Job drawing, mm, ordinate dimensions from the low corner. One solid piece. A direction names the side the tool comes from. Give positions to 0.01 mm unless a question says otherwise; leave off trailing zeros. Order: outer loops, then holes, each group sorted by start corner. A loop starts at its lowest first (then second) coordinate and runs counter-clockwise, first axis right, second up. Notation, with made-up numbers: (-31.5, 31) -> (-0.5, 31) arc R14 ccw to (-0.5, 40) -> close; hole circle Ø3 at (-37.5, 29). An arc over 180 degrees is marked (long way). Write item = value, one per line. Start each with the question number.
(1) Which spindle directions (+Z, -Z, +X, -X, +Y, -Y) get a long thin tool onto all of the face, cutting with end or side? Do the marked faces 1 and 2. Say none if no direction does.
(2) Probe line 1 along X through (y, z) = (4.75, 4); line 2 along Z through (x, y) = (5.5, 13); line 3 along Y through (x, z) = (1.5, 10.5). List the from-to ranges inside material, lowest first. Write a range as from..to.
(3) Saw through at D-D, the plane z = 21.75. List the corners of the cut face in (x, y), then the cut area to 3 significant figures.
(4) Saw through at A-A, the plane z = 13. List the corners of the cut face in (x, y) (3 decimals).
(5) Flat gauge pins, fed straight in: pin 1 (3 mm diameter, centred on y = 13, z = 21.5, fed in from -X); pin 2 (10 mm diameter, centred on x = 8.5, z = 15, fed in from -Y); pin 3 (2 mm diameter, centred on x = 3.5, z = 11.5, fed in from +Y); pin 4 (1.5 mm diameter, centred on x = 4, z = 6, fed in from +Y). Where does each tip first touch, or does it go through?
(6) Saw through at C-C, the plane x = 11.25. List the corners of the cut face in (y, z), then the cut area to 3 significant figures.
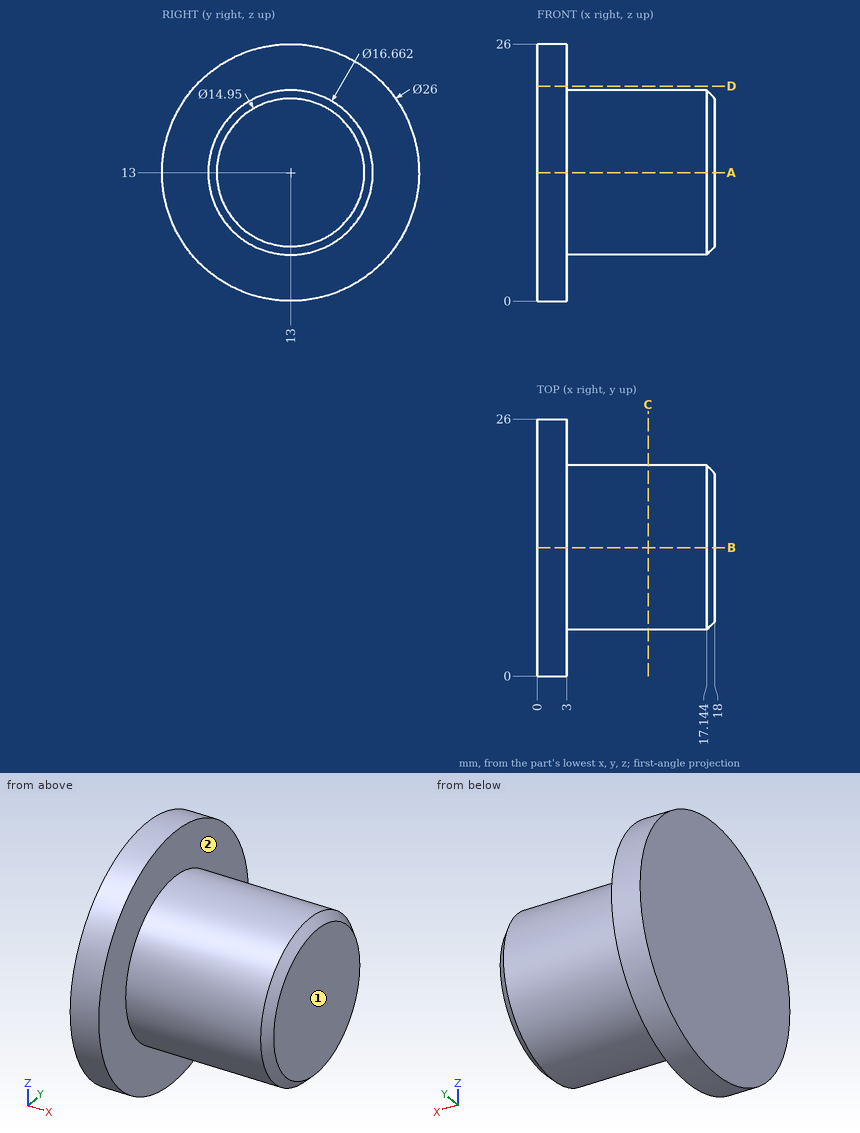
Results list:
q1.face_1 = +Z, -Z, +X, +Y, -Y
q1.face_2 = +X
q2.line_1 = 0..3
q2.line_2 = 4.67..21.33
q2.line_3 = 0.24..25.76
q3.outline = (0, 3.39) -> (3, 3.39) -> (3, 22.61) -> (0, 22.61) -> close
q3.area = 57.7 mm^2
q4.outline = (0, 0) -> (3, 0) -> (3, 4.669) -> (17.144, 4.669) -> (18, 5.525) -> (18, 20.475) -> (17.144, 21.331) -> (3, 21.331) -> (3, 26) -> (0, 26) -> close
q5.pin_1 = 0
q5.pin_2 = 4.67
q5.pin_3 = 25.98
q5.pin_4 = 18.51
q6.outline = circle Ø16.66 at (13, 13)
q6.area = 218 mm^2
